```python
from build123d import *

# Parameters (mm, degrees)
SKETCH1_R           = 3.225
BOSS_EXTRUDE1_DEPTH = 1.2


with BuildPart() as part:
    # Sketch1 → Boss-Extrude1 (new body)
    with BuildSketch(Plane.XY):
        with BuildLine():
            ThreePointArc((4.65, 25.4), (0, 30.05), (-4.65, 25.4))
            Line((-4.65, 25.4), (-4.65, 23))
            ThreePointArc((-4.65, 23), (-5.235786438, 21.585786438), (-6.65, 21))
            Line((-6.65, 21), (-8.759132098, 21))
            Line((-8.759132098, 21), (-21, 21))
            Line((-21, 21), (-21, 7.133487824))
            Line((-21, 7.133487824), (-21, 6.65))
            ThreePointArc((-21, 6.65), (-21.585786438, 5.235786438), (-23, 4.65))
            Line((-23, 4.65), (-25.4, 4.65))
            ThreePointArc((-25.4, 4.65), (-30.05, 0), (-25.4, -4.65))
            Line((-25.4, -4.65), (-23, -4.65))
            ThreePointArc((-23, -4.65), (-21.585786438, -5.235786438), (-21, -6.65))
            Line((-21, -6.65), (-21, -8.759132098))
            Line((-21, -8.759132098), (-21, -21))
            Line((-21, -21), (-7.133487824, -21))
            Line((-7.133487824, -21), (-6.65, -21))
            ThreePointArc((-6.65, -21), (-5.235786438, -21.585786438), (-4.65, -23))
            Line((-4.65, -23), (-4.65, -25.4))
            ThreePointArc((-4.65, -25.4), (0, -30.05), (4.65, -25.4))
            Line((4.65, -25.4), (4.65, -23))
            ThreePointArc((4.65, -23), (5.235786438, -21.585786438), (6.65, -21))
            Line((6.65, -21), (8.759132098, -21))
            Line((8.759132098, -21), (21, -21))
            Line((21, -21), (21, -7.133487824))
            Line((21, -7.133487824), (21, -6.65))
            ThreePointArc((21, -6.65), (21.585786438, -5.235786438), (23, -4.65))
            Line((23, -4.65), (25.4, -4.65))
            ThreePointArc((25.4, -4.65), (30.05, 0), (25.4, 4.65))
            Line((25.4, 4.65), (23, 4.65))
            ThreePointArc((23, 4.65), (21.585786438, 5.235786438), (21, 6.65))
            Line((21, 6.65), (21, 8.759132098))
            Line((21, 8.759132098), (21, 21))
            Line((21, 21), (7.133487824, 21))
            Line((7.133487824, 21), (6.65, 21))
            ThreePointArc((6.65, 21), (5.235786438, 21.585786438), (4.65, 23))
            Line((4.65, 23), (4.65, 25.4))
        make_face()
        with Locations((0, -25.4)):
            Circle(SKETCH1_R, mode=Mode.SUBTRACT)
        with Locations((25.4, 0)):
            Circle(SKETCH1_R, mode=Mode.SUBTRACT)
        with Locations((-25.4, 0)):
            Circle(SKETCH1_R, mode=Mode.SUBTRACT)
        with Locations((0, 25.4)):
            Circle(SKETCH1_R, mode=Mode.SUBTRACT)
    extrude(amount=BOSS_EXTRUDE1_DEPTH)


solid = part.part
```
Model file for the job. Use its own axes, mm. Give positions to 0.01 mm unless a question says otherwise; leave off trailing zeros. Order: outer loops, then holes, each group sorted by start corner. A loop starts at its lowest first (then second) coordinate and runs counter-clockwise, first axis right, second up.
1) Saw through at B-B, the plane z = 0.6. Count the separate pieces of the cut face and the enclosed holes in it, then the cut area to 3 significant figures.
2) Saw through at D-D, the plane x = 10.5. Write the cut outline in (y, z).
3) Mould opens along Y. For faces 1 (the cylindrical face through (0.1, 30.05, 0.59)), 2 (the cylindrical face through (22.18, 0.14, 0.59)), 3 (the cylindrical face through (-30.05, 0.1, 0.59)) say: +Y half, -Y half, draft (parallel to the pull), parting line (faces both ways), or undercut.
4) Pin check, flat tips, straight feed: pin 1 (6 mm diameter, centred on x = 25.4, y = 0, fed in from +Z); pin 2 (0.6 mm diameter, centred on x = 13.5, z = 0.5, fed in from -Y); pin 3 (0.6 mm diameter, centred on x = 17, z = 0.5, fed in from +Y). Stop position of each tip, or through.
5) Wall check: probe 1 along Y at (x, z) = (0, 0.65) (3 decimals); probe 2 along Y at (x, z) = (25.4, 0.6) (3 decimals); probe 3 along X at (y, z) = (13, 0.5). Give the ranges that are in metal, low to high.
6) Saw through at A-A, the plane x = 0. Write the cut outline in (y, z) (3 decimals), then the cut area to 3 significant figures.
Computed:
1. separate pieces: 1
1. enclosed holes: 4
1. area: 1,940 mm2
2. outline: (-21, 0) - (21, 0) - (21, 1.2) - (-21, 1.2) - close
3. face 1: +Y half
3. face 2: undercut
3. face 3: parting line
4. pin 1: passes through
4. pin 2: stops at y = -21
4. pin 3: stops at y = 21
5. probe 1: y = -30.05 to -28.625, -22.175 to 22.175, 28.625 to 30.05
5. probe 2: y = -4.65 to -3.225, 3.225 to 4.65
5. probe 3: x = -21 to 21
6. outline: (-30.05, 0) - (-28.625, 0) - (-28.625, 1.2) - (-30.05, 1.2) - close; (-22.175, 0) - (22.175, 0) - (22.175, 1.2) - (-22.175, 1.2) - close; (28.625, 0) - (30.05, 0) - (30.05, 1.2) - (28.625, 1.2) - close
6. area: 56.6 mm2
